from build123d import *

# Parameters (mm, degrees)
F0_R     = 18
F0_R_2   = 15
F1_DEPTH = 25
F2_SIZE2 = 1.091514
F2_SIZE  = 24.99999
F3_W     = 11.1970370635
F3_H     = 2.7507020859
F3_W_2   = 2.8398953145
F3_H_2   = 11.1970370635
F3_H_3   = 3.1587614212
F3_W_3   = 2.980374964
F4_DEPTH = 1


# Not quite as in the source:
# - a fillet or chamfer is up to 0.001 mm smaller than in the source, because OpenCascade refuses the exact size


with BuildPart() as f1:
    # F0 (on Top) → F1 (new body)
    with BuildSketch(Plane.XY):
        Circle(F0_R)
        Circle(F0_R_2, mode=Mode.SUBTRACT)
    extrude(amount=F1_DEPTH)

    # F2 (size 25 and 1.0915235727 in the source; OpenCascade refuses exactly that, so slightly less here)
    f2_edges = [f1.edges().sort_by_distance(p)[0] for p in [
        (-15, 0, 25),
    ]]
    f2_side = f1.faces().sort_by_distance((-15, 0, 12.5))[0]
    chamfer(f2_edges, length=F2_SIZE, length2=F2_SIZE2, reference=f2_side)

    # F3 (on Top) → F4 (join)
    with BuildSketch(Plane.XY):
        with Locations((-9.9286013283, 2.9547317536)):
            Rectangle(F3_W, F3_H)
        with Locations((-9.9286013283, -2.9547317536)):
            Rectangle(F3_W, F3_H)
        with Locations((2.9101351392, 9.9286013283)):
            Rectangle(F3_W_2, F3_H_2)
        with Locations((-2.9101351392, 9.9286013283)):
            Rectangle(F3_W_2, F3_H_2)
        with Locations((9.9286013283, 2.9547317536)):
            Rectangle(F3_W, F3_H)
        with Locations((9.9286013283, -2.9547317536)):
            Rectangle(F3_W, F3_H)
        with Locations((2.9101351392, -9.9286013283)):
            Rectangle(F3_W_2, F3_H_2)
        with Locations((-2.9101351392, -9.9286013283)):
            Rectangle(F3_W_2, F3_H_2)
        with Locations((2.9101351392, 2.9547317536)):
            Rectangle(F3_W_2, F3_H)
        with Locations((-2.9101351392, 2.9547317536)):
            Rectangle(F3_W_2, F3_H)
        with Locations((-2.9101351392, 0)):
            Rectangle(F3_W_2, F3_H_3)
        with Locations((-2.9101351392, -2.9547317536)):
            Rectangle(F3_W_2, F3_H)
        with Locations((0, -2.9547317536)):
            Rectangle(F3_W_3, F3_H)
        with Locations((2.9101351392, -2.9547317536)):
            Rectangle(F3_W_2, F3_H)
        with Locations((2.9101351392, 0)):
            Rectangle(F3_W_2, F3_H_3)
        with Locations((0, 2.9547317536)):
            Rectangle(F3_W_3, F3_H)
        Rectangle(F3_W_3, F3_H_3)
    extrude(amount=F4_DEPTH)


solid = f1.part
Part model, mm, in its own coordinate system. A direction names the side the tool comes from. Round coordinates to 2 decimals unless told otherwise and drop trailing zeros. Return JSON: item names as keys, results as strings. Group by question number.
(1) Pin check, flat tips, straight feed: pin 1 Ø0.5 at (y, z) = (-9.5, 0.5) entering from +X; pin 2 Ø0.8 at (x, z) = (7.5, 0.5) entering from +Y; pin 3 Ø1.1 at (x, z) = (7.5, 0.5) entering from -Y. Stop position of each tip, or through.
(2) Saw through at A-A on x = 0. Count the separate pieces of the cut face and the enclosed holes in it, then the cut area to 3 significant figures.
(3) Drill centre lines: probe 1 along X at (y, z) = (-4.5, 14); probe 2 along Z at (x, y) = (-4, -13.5); probe 3 along X at (y, z) = (-1, 6). Where is each one in solid material? Low to high.
(4) Which spindle directions (+Z, -Z, +X, -X, +Y, -Y) get a long thin tool onto all of the face, cutting with end or side? Do faces 4 (the face through (0, 0, 1)), 5 (the face through (9.6, 1.579, 0.5)). Say none if no direction does.
(5) Two-plate mould, pull along X, no slides. Class faces 1 (the face through (-2.343, 17.847, 12.325)), 2 (the face through (1.49, -9.7, 0.5)), 3 (the face through (0, 0, 0)): +X half, -X half, draft (parallel to the pull), parting line (faces both ways), or undercut.
Returned:
{
 "1": {"pin 1": "x = 15.44", "pin 2": "y = 16.54", "pin 3": "y = -16.6"},
 "2": {"separate pieces": "3", "enclosed holes": "0", "area": "131 mm²"},
 "3": {"probe 1": "-17.43 to -14.95, 14.95 to 17.43", "probe 2": "0 to 1", "probe 3": "-17.97 to -15.23, 15.23 to 17.97"},
 "4": {"face 4": "+Z", "face 5": "+Z, -Z"},
 "5": {"face 1": "parting line", "face 2": "undercut", "face 3": "draft"}
}
